Read the model definition and answer for the solid it produces. Units are mm, in the model's axes. Face numbers are marked on the shaded views. A direction names the side the tool comes from. Coordinates: 2 decimals unless noted, no trailing zeros. Write each loop counter-clockwise with the first axis right and the second up, starting at its lowest first coordinate (ties: lowest second). Pieces come first, ordered by that corner, then holes.
(1) The part is cut by section C-C, the plane x = 38.7. Determine the outline of the cut face in (y, z).
(2) The part is cut by section A-A, the plane x = 13. Determine the outline of the cut face in (y, z).
(3) The part is cut by section B-B, the plane y = -24. Determine the outline of the cut face in (x, z), and give its area (3 significant figures).
(4) Determine the mould class of the marked faces 1, 2, 3 and 4 for opening direction X: pulls with the +X half, pulls with the -X half, needs draft (parallel to the pull), parting line crosses it, or undercut.
(5) The part is cut by section D-D, the plane x = -46. Determine the outline of the cut face in (y, z).
(6) Which of the six approach directions +Z, -Z, +X, -X, +Y, -Y give full straight-line access (tool end or side, diameter ignored) to the marked faces 5 and 6?
(7) Straight lines are drawn through the part: line 1 along Y through (x, z) = (-41.3, 1.15); line 2 along Y through (x, z) = (26.5, 31); line 3 along X through (y, z) = (-34.5, 6.5). For each, find the intervals that lie inside material, in ascending order.
```python
from build123d import *

# Parameters (mm, degrees)
SKETCH_W        = 112.6
SKETCH_H        = 34
PAD_DEPTH       = 41
SKETCH005_W     = 106.6
SKETCH005_H     = 35
POCKET_DEPTH    = 31
SKETCH007_R     = 13
POCKET001_DEPTH = 41.001
SKETCH006_R     = 1.75
SKETCH006_R_2   = 15
POCKET002_DEPTH = 5
SKETCH008_R     = 12.575466
POCKET003_DEPTH = 112.601


with BuildPart() as part:
    # Sketch → Pad (new body)
    with BuildSketch(Plane.XZ):
        with Locations((0, 17)):
            Rectangle(SKETCH_W, SKETCH_H)
    extrude(amount=PAD_DEPTH)

    # Sketch005 → Pocket (cut)
    with BuildSketch(Plane(origin=(0, 0, 34), x_dir=(-1, 0, 0), z_dir=(0, 0, 1))):
        with Locations((0, 20.5)):
            Rectangle(SKETCH005_W, SKETCH005_H)
    extrude(amount=-POCKET_DEPTH, mode=Mode.SUBTRACT)

    # Sketch007 → Pocket001 (cut, through all)
    with BuildSketch(Plane.XZ.offset(41)):
        with Locations((-23.3, 17.5)):
            Circle(SKETCH007_R)
        with Locations((7.7, 17.5)):
            Circle(SKETCH007_R)
        with Locations((38.7, 17.5)):
            Circle(SKETCH007_R)
        with BuildLine():
            ThreePointArc((-42.3, 26), (-47.3, 31), (-52.3, 26))
            Line((-52.3, 26), (-52.3, 8.000019))
            ThreePointArc((-52.3, 8.000019), (-47.3, 3), (-42.3, 8.000019))
            Line((-42.3, 26), (-42.3, 8.000019))
        make_face()
    extrude(amount=-POCKET001_DEPTH, mode=Mode.SUBTRACT)

    # Sketch006 → Pocket002 (cut)
    with BuildSketch(Plane(origin=(0, 0, 0), x_dir=(1, 0, 0), z_dir=(0, 0, -1))):
        with Locations((-41.3, 30)):
            Circle(SKETCH006_R)
        with Locations((38.7, 30)):
            Circle(SKETCH006_R)
        with Locations((-41.3, 5)):
            Circle(SKETCH006_R)
        with Locations((38.7, 5)):
            Circle(SKETCH006_R)
        with Locations((-20, 20)):
            Circle(SKETCH006_R_2)
        with Locations((20, 20)):
            Circle(SKETCH006_R_2)
    extrude(amount=-POCKET002_DEPTH, mode=Mode.SUBTRACT)

    # Sketch008 → Pocket003 (cut, through all)
    with BuildSketch(Plane(origin=(56.3, 0, 0), x_dir=(0, 0, 1), z_dir=(1, 0, 0))):
        with Locations((17.195639, 20)):
            Circle(SKETCH008_R)
    extrude(amount=-POCKET003_DEPTH, mode=Mode.SUBTRACT)


solid = part.part
```
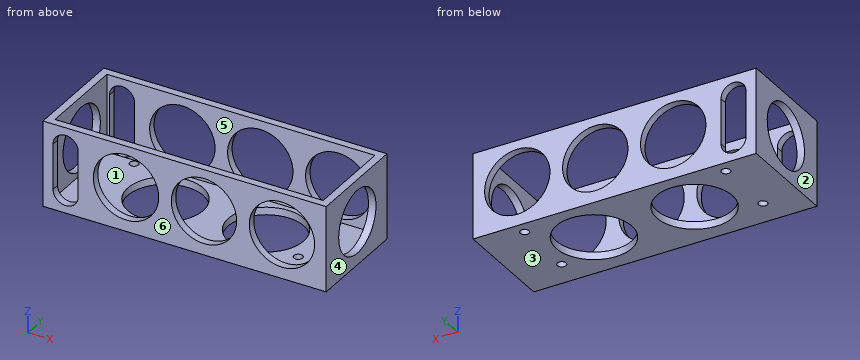
Computed:
1. outline: (-41, 0) - (-31.75, 0) - (-31.75, 3) - (-38, 3) - (-38, 4.5) - (-41, 4.5) - close; (-41, 30.5) - (-38, 30.5) - (-38, 34) - (-41, 34) - close; (-28.25, 0) - (-6.75, 0) - (-6.75, 3) - (-28.25, 3) - close; (-3.25, 0) - (0, 0) - (0, 4.5) - (-3, 4.5) - (-3, 3) - (-3.25, 3) - close; (-3, 30.5) - (0, 30.5) - (0, 34) - (-3, 34) - close
2. outline: (-41, 0) - (-33.27, 0) - (-33.27, 3) - (-38, 3) - (-38, 5.63) - (-41, 5.63) - close; (-41, 29.37) - (-38, 29.37) - (-38, 34) - (-41, 34) - close; (-6.73, 0) - (0, 0) - (0, 5.63) - (-3, 5.63) - (-3, 3) - (-6.73, 3) - close; (-3, 29.37) - (0, 29.37) - (0, 34) - (-3, 34) - close
3. outline: (-56.3, 0) - (-34.46, 0) - (-34.46, 3) - (-53.3, 3) - (-53.3, 5.27) - (-56.3, 5.27) - close; (-56.3, 29.12) - (-53.3, 29.12) - (-53.3, 34) - (-56.3, 34) - close; (-5.54, 0) - (5.54, 0) - (5.54, 3) - (-5.54, 3) - close; (34.46, 0) - (56.3, 0) - (56.3, 5.27) - (53.3, 5.27) - (53.3, 3) - (34.46, 3) - close; (53.3, 29.12) - (56.3, 29.12) - (56.3, 34) - (53.3, 34) - close
3. area: 207 mm2
4. face 1: undercut
4. face 2: pulls with the -X half
4. face 3: needs draft
4. face 4: pulls with the +X half
5. outline: (-41, 0) - (0, 0) - (0, 3.17) - (-3, 3.17) - (-3, 3) - (-38, 3) - (-38, 3.17) - (-41, 3.17) - close; (-41, 30.83) - (-38, 30.83) - (-38, 34) - (-41, 34) - close; (-3, 30.83) - (0, 30.83) - (0, 34) - (-3, 34) - close
6. face 5: +Z
6. face 6: +Z, -Z, +X, -X, -Y
7. line 1: y = -41 to -31.75, -28.25 to -6.75, -3.25 to 0
7. line 2: y = -41 to -38, -3 to 0
7. line 3: x = -56.3 to -53.3, 53.3 to 56.3
